```python
from build123d import *

# Parameters (mm, degrees)
F1_R      = 1.65
F2_DEPTH  = 6
F3_R      = 3.75
F4_DEPTH  = 12.001
F5_R      = 6
F5_R_2    = 1.25
F6_DEPTH  = 6
F7_SIZE2  = 4
F7_SIZE   = 2
F8_R      = 6
F9_DEPTH  = 12
F9_TAPER  = 10
F10_R     = 2.15
F11_DEPTH = 12
F12_R     = 3
F13_DEPTH = 3
F14_R     = 3
F15_DEPTH = 3


with BuildPart() as f2:
    # F1 (on Front) → F2 (new body)
    with BuildSketch(Plane.XZ):
        with BuildLine():
            Line((15, 0), (15, 4))
            ThreePointArc((15, 4), (14.1725596506, 6.7549493575), (11.9641016151, 8.5980762114))
            Line((11.9641016151, 8.5980762114), (4.9409269852, 11.5980762114))
            ThreePointArc((4.9409269852, 11.5980762114), (3.9792272214, 11.8984885963), (2.9768253701, 12))
            Line((2.9768253701, 12), (0, 12))
            Line((0, 12), (-2.9768253701, 12))
            ThreePointArc((-2.9768253701, 12), (-3.9792272214, 11.8984885963), (-4.9409269852, 11.5980762114))
            Line((-4.9409269852, 11.5980762114), (-11.9641016151, 8.5980762114))
            ThreePointArc((-11.9641016151, 8.5980762114), (-14.1725596506, 6.7549493575), (-15, 4))
            Line((-15, 4), (-15, 0))
            Line((-15, 0), (0, 0))
            Line((0, 0), (15, 0))
        make_face()
        with Locations((-10, 4)):
            Circle(F1_R, mode=Mode.SUBTRACT)
        with Locations((10, 4)):
            Circle(F1_R, mode=Mode.SUBTRACT)
    extrude(amount=-F2_DEPTH)

    # F3 (on face) → F4 (cut, through all)
    with BuildSketch(Plane.XY.offset(12)):
        Circle(F3_R)
    extrude(amount=-F4_DEPTH, mode=Mode.SUBTRACT)



with BuildPart() as f6:
    # F5 (on Top) → F6 (new body)
    with BuildSketch(Plane.XY):
        Circle(F5_R)
        Circle(F5_R_2, mode=Mode.SUBTRACT)
    extrude(amount=F6_DEPTH)

    # F7
    f7_edges = [f6.edges().sort_by_distance(p)[0] for p in [
        (-1.25, 0, 0),
    ]]
    f7_side = f6.faces().sort_by_distance((-5.830294, 0, 0))[0]
    chamfer(f7_edges, length=F7_SIZE, length2=F7_SIZE2, reference=f7_side)


with BuildPart() as f2_1:
    add(f2.part)

    add(f6.part)  # F9 merges F6
    # F8 (on face) → F9 (join)
    with BuildSketch(Plane.XY.offset(6)):
        Circle(F8_R)
    extrude(amount=F9_DEPTH, taper=F9_TAPER)

    # F10 (on face) → F11 (cut)
    with BuildSketch(Plane.XY.offset(18)):
        Circle(F10_R)
    extrude(amount=-F11_DEPTH, mode=Mode.SUBTRACT)

    # F12 (on face) → F13 (cut)
    with BuildSketch(Plane.XZ):
        with Locations((-10, 4)):
            Circle(F12_R)
    extrude(amount=-F13_DEPTH, mode=Mode.SUBTRACT)

    # F14 (on face) → F15 (cut)
    with BuildSketch(Plane.XZ):
        with Locations((10, 4)):
            Circle(F14_R)
    extrude(amount=-F15_DEPTH, mode=Mode.SUBTRACT)


solid = f2_1.part
```
Model file for the job. Use its own axes, mm. A direction names the side the tool comes from. Give positions to 0.01 mm unless a question says otherwise; leave off trailing zeros. Write each loop counter-clockwise with the first axis right and the second up, starting at its lowest first coordinate (ties: lowest second). Pieces come first, ordered by that corner, then holes. Notation, with made-up numbers: M 74,88 L 91,88 A33 cw 91,125 Z; hole C 56.5,70.5 d5. An arc over 180 degrees is marked long. Use a Markdown table: item, result.
1) Pin check, flat tips, straight feed: pin 1 (2 mm diameter, centred on x = 1, z = 15, fed in from +Y); pin 2 (2 mm diameter, centred on y = -4.5, z = 7, fed in from -X); pin 3 (3 mm diameter, centred on x = 0, y = 0, fed in from +Z). Stop position of each tip, or through.
Responses:
| item | result |
|---|---|
| pin 1 | stops at y = 4.54 |
| pin 2 | stops at x = -4.69 |
| pin 3 | stops at z = 6 |
2) Cut at C-C (z = 11.25). List the corners of the cut face in (x, y), and give its area (3 significant figures).
Responses:
| item | result |
|---|---|
| outline | M -5.76,0 L -5.07,0 A5.07 ccw 5.07,0 L 5.76,0 L 5.76,6 L -5.76,6 Z; hole C 0,0 d4.3 |
| area | 95.0 mm2 |
3) Tool access for faces 1 (the cylindrical face through (-12.4, 1.5, 2.2)), 2 (the flat face through (1, -1, 6)), 3 (the cylindrical face through (4.212, 4.532, 11.845)), 4 (the cylindrical face through (-8.476, 4.479, 3.368)): list every direction of +Z, -Z, +X, -X, +Y, -Y with a clear straight run to the whole face (end or side of a thin tool).
Responses:
| item | result |
|---|---|
| face 1 | -Y |
| face 2 | +Z |
| face 3 | +Z, +X, +Y |
| face 4 | +Y, -Y |
4) Cut at D-D (y = 1.75). Give the number of separate pieces and of enclosed holes in the cut face, and give its area (3 significant figures).
Responses:
| item | result |
|---|---|
| separate pieces | 1 |
| enclosed holes | 2 |
| area | 256 mm2 |
5) Pull direction Z, two halves, no side cores. Call faces 5 (the flat face through (-8.7, 3, 2.7)), 6 (the conical face through (2.17, -4.16, 13.42)), 7 (the flat face through (11.3, 3, 2.7)), 8 (the flat face through (0, 6, 5)): +Z half, -Z half, draft (parallel to the pull), parting line (faces both ways), or undercut.
Responses:
| item | result |
|---|---|
| face 5 | undercut |
| face 6 | +Z half |
| face 7 | undercut |
| face 8 | draft |
6) Drill centre lines: line 1 (Y direction, x = 0, z = 5.05); line 2 (X direction, y = 5, z = 4.25); line 3 (Z direction, x = -2.75, y = 4.5). Where is each one in solid material? Low to high. Write a range as from..to.
Responses:
| item | result |
|---|---|
| line 1 | y = -6..-1.25, 1.25..6 |
| line 2 | x = -14.99..-11.63, -8.37..8.37, 11.63..14.99 |
| line 3 | z = 0..12 |
7) Cut at B-B (z = 2.75). List the corners of the cut face in (x, y) (3 decimals).
Responses:
| item | result |
|---|---|
| outline | M -15,0 L -12.727,0 L -12.727,3 L -11.077,3 L -11.077,6 L -15,6 Z; M -8.923,3 L -7.273,3 L -7.273,0 L -6,0 A6 ccw 6,0 L 7.273,0 L 7.273,3 L 8.923,3 L 8.923,6 L -8.923,6 Z; M 11.077,3 L 12.727,3 L 12.727,0 L 15,0 L 15,6 L 11.077,6 Z; hole C 0,0 d3.75 |
8) Cut at A-A (x = 0). List the corners of the cut face in (y, z), and give its area (3 significant figures).
Responses:
| item | result |
|---|---|
| outline | M -6,0 L -3.25,0 L -1.25,4 L -1.25,6 L -2.15,6 L -2.15,18 L -3.88,18 L -6,6 Z; M 1.25,4 L 3.25,0 L 6,0 L 6,12 L 4.94,12 L 3.88,18 L 2.15,18 L 2.15,6 L 1.25,6 Z |
| area | 119 mm2 |
